Input: part model. Units: mm. Frame: model coordinates. Face numbers are marked on the shaded views. A direction names the side the tool comes from. Coordinates: 2 decimals unless noted, no trailing zeros. Write each loop counter-clockwise with the first axis right and the second up, starting at its lowest first coordinate (ties: lowest second). Pieces come first, ordered by that corner, then holes. Notation, with made-up numbers: M 87,-26.75 L 98,-26.75 A16 cw 98,2.25 Z; hole C -21.75,47 d9. An arc over 180 degrees is marked long. Use one line per item in the form item = value.
from build123d import *

# Parameters (mm, degrees)
F0_R     = 2
F1_DEPTH = 4
F2_W     = 30
F2_H     = 2.5
F3_DEPTH = 13
F4_R     = 1.75
F4_R_2   = 2
F5_DEPTH = 25


with BuildPart() as f1:
    # F0 (on Front) → F1 (new body)
    with BuildSketch(Plane.XZ):
        Polygon((11, -15), (15, -15), (15, 15), (-15, 15), (-15, -15), (-11, -15), (-11, -1), (-7, -1), (-7, -15), (7, -15), (7, -1), (11, -1), align=None)
        with Locations((0, -3.5)):
            Circle(F0_R, mode=Mode.SUBTRACT)
        with Locations((-4.5, 5.5)):
            Circle(F0_R, mode=Mode.SUBTRACT)
        with Locations((4.5, 5.5)):
            Circle(F0_R, mode=Mode.SUBTRACT)
    extrude(amount=F1_DEPTH)

    # F2 (on face) → F3 (join)
    with BuildSketch(Plane.XZ.offset(4)):
        with Locations((0, 9.75)):
            Rectangle(F2_W, F2_H)
    extrude(amount=F3_DEPTH)

    # F4 (on face) → F5 (cut)
    with BuildSketch(Plane(origin=(0, 0, 8.5), x_dir=(1, 0, 0), z_dir=(0, 0, -1))):
        with Locations((-8.75, 11)):
            Circle(F4_R)
        with Locations((0, 11)):
            Circle(F4_R_2)
        with Locations((8.75, 11)):
            Circle(F4_R)
    extrude(amount=-F5_DEPTH, mode=Mode.SUBTRACT)


solid = f1.part
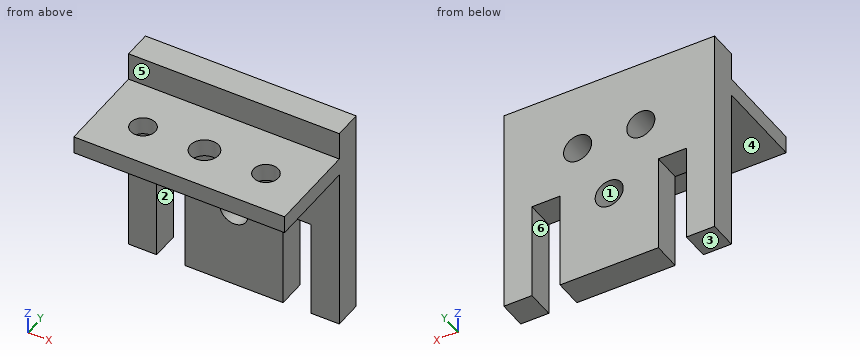
(1) Section query C-C on x = 0. Return the cut outline in (y, z), plus the area to 4 significant figures.
Computed:
outline = M -17,8.5 L -13,8.5 L -13,11 L -17,11 Z; M -9,8.5 L -4,8.5 L -4,-1.5 L 0,-1.5 L 0,15 L -4,15 L -4,11 L -9,11 Z; M -4,-15 L 0,-15 L 0,-5.5 L -4,-5.5 Z
area = 126.5 mm^2
(2) Section query D-D on z = -3.5. Return the cut outline in (x, y), plus the area to 3 significant figures.
Computed:
outline = M -15,-4 L -11,-4 L -11,0 L -15,0 Z; M -7,-4 L -2,-4 L -2,0 L -7,0 Z; M 2,-4 L 7,-4 L 7,0 L 2,0 Z; M 11,-4 L 15,-4 L 15,0 L 11,0 Z
area = 72.0 mm^2
(3) First-contact query: pin 1 Ø1 at (x, y) = (0, -14) entering from +Z; pin 2 Ø1.5 at (x, y) = (-6, -9.5) entering from -Z; pin 3 Ø2 at (x, y) = (-9.5, -1) entering from -Z. Flat tips, straight axial feed; report the tip coordinate or a pass-through.
Computed:
pin_1 = 11
pin_2 = 8.5
pin_3 = -1
(4) Set-up query: the marked faces 4, 5 and 6. Return all of +Z, -Z, +X, -X, +Y, -Y with unobstructed straight access to the full face (end or side cutting, diameter ignored); none if empty.
Computed:
face_4 = -Z, +X, -X, -Y
face_5 = +Z, +X, -X, -Y
face_6 = -Z, +Y, -Y
(5) Section query B-B on z = -13. Return the cut outline in (x, y), plus the area to 3 significant figures.
Computed:
outline = M -15,-4 L -11,-4 L -11,0 L -15,0 Z; M -7,-4 L 7,-4 L 7,0 L -7,0 Z; M 11,-4 L 15,-4 L 15,0 L 11,0 Z
area = 88.0 mm^2
(6) Section query A-A on x = 4.5. Return the cut outline in (y, z).
Computed:
outline = M -17,8.5 L -4,8.5 L -4,7.5 L 0,7.5 L 0,15 L -4,15 L -4,11 L -17,11 Z; M -4,-15 L 0,-15 L 0,3.5 L -4,3.5 Z
(7) Pull-direction query (Z, two-part tool) for the marked faces 1, 2 and 3; classes: pulls with the +Z half, pulls with the -Z half, needs draft (parallel to the pull), parting line crosses it, or undercut.
Computed:
face_1 = undercut
face_2 = needs draft
face_3 = pulls with the -Z half
(8) Line query: probe 1 along X at (y, z) = (-11, 9.85); probe 2 along Z at (x, y) = (-4.5, -1.6); probe 3 along Z at (x, y) = (0, -3.05). Output: solid intervals per line, ascending.
Computed:
probe_1 = -15 to -10.5, -7 to -2, 2 to 7, 10.5 to 15
probe_2 = -15 to 3.5, 7.5 to 15
probe_3 = -15 to -5.5, -1.5 to 15
